Can you work these out from the model? Positions are in its coordinate system, mm. A direction names the side the tool comes from. Give positions to 0.01 mm unless a question says otherwise; leave off trailing zeros. Loops run counter-clockwise (first coordinate to the right, second up) from the corner with the lowest first, then second, coordinate; pieces in that order, holes last. Notation, with made-up numbers: (84.25, 3) - (98.25, 3) arc R16 ccw to (98.25, 15) - close; hole circle Ø3 at (10, 80.5). An arc over 180 degrees is marked (long way). Answer as a JSON object with one key per item and string values. Group by question number.
Item 1: Suppose I cut it at D-D on z = -18.5. Write out the boundary of the cut face in (x, y).
Item 2: Thinking about a two-plate mould opening in Y: for faces 3 (the flat face through (50, 16.8, -5)), 4 (the cylindrical face through (50.089, 9.937, -2.367)), 5 (the flat face through (50, 18, -9.525)), which applies, pulls with the +Y half, pulls with the -Y half, needs draft (parallel to the pull), parting line crosses it, or undercut?
Item 3: Please list where these lines run through material, in increasing order: L1, parallel to X at y = 10, z = -5; L2, parallel to Y at x = 23.5, z = -5; L3, parallel to Z at x = 82.55, y = 13.5.
Item 4: Suppose I cut it at B-B on x = 23.5. Write out the boundary of the cut face in (y, z) (3 decimals), and give its area (3 significant figures).
Item 5: Which directions (+Z, -Z, +X, -X, +Y, -Y) give clear straight access to the entire face, cutting with the end or side of a thin tool? Please do faces 1 (the flat face through (50, 3.2, -5)), 2 (the cylindrical face through (84.075, 10.095, -4.13)).
Item 6: Suppose I cut it at C-C on y = 15. Write out the boundary of the cut face in (x, z), and give its area (3 significant figures).
Item 7: Will these pins go through, and if not, where does the flat tip stop? pin 1 (2 mm diameter, centred on x = 54, y = 10, fed in from +Z); pin 2 (1.6 mm diameter, centred on x = 36.5, y = 18, fed in from +Z) (3 decimals); pin 3 (10.5 mm diameter, centred on x = 29, z = -4, fed in from +Y).
from build123d import *

# Parameters (mm, degrees)
BOSS_EXTRUDE1_DEPTH = 101.6
CUT_EXTRUDE2_DEPTH  = 101.6
SKETCH5_R           = 1.651
CUT_EXTRUDE3_DEPTH  = 13.5992
FILLET1_R           = 2.54


with BuildPart() as part:
    # Sketch1 → Boss-Extrude1 (new body)
    with BuildSketch(Plane(origin=(0, 0, 0), x_dir=(0, 0, -1), z_dir=(1, 0, 0))):
        with BuildLine():
            Line((0, 16.7996), (0, 3.2004))
            Line((0, 3.2004), (9.525, 3.2004))
            Line((9.525, 3.2004), (9.525, 0))
            Line((9.525, 0), (9.672001208, 0))
            ThreePointArc((9.672001208, 0), (12.1043061, 0.647018058), (13.89365381, 2.417039025))
            Line((13.89365381, 2.417039025), (24.215623453, 20))
            Line((24.215623453, 20), (9.525, 20))
            Line((9.525, 20), (9.525, 16.7996))
            Line((9.525, 16.7996), (0, 16.7996))
        make_face()
    extrude(amount=BOSS_EXTRUDE1_DEPTH)

    # Sketch4 → Cut-Extrude2 (cut)
    with BuildSketch(Plane.ZY):
        with BuildLine():
            Line((0, 13.526281186), (0, 6.473718814))
            ThreePointArc((0, 6.473718814), (-2.36728, 10), (0, 13.526281186))
        make_face()
    extrude(amount=-CUT_EXTRUDE2_DEPTH, mode=Mode.SUBTRACT)

    # Sketch5 → Cut-Extrude3 (cut)
    with BuildSketch(Plane(origin=(0, 16.7996, 0), x_dir=(1, 0, 0), z_dir=(0, 1, 0))):
        with Locations((19.05, 4.7625)):
            Circle(SKETCH5_R)
        with Locations((82.55, 4.7625)):
            Circle(SKETCH5_R)
    extrude(amount=-CUT_EXTRUDE3_DEPTH, mode=Mode.SUBTRACT)

    # Fillet1
    fillet1_edges = [part.edges().sort_by_distance(p)[0] for p in [
        (50.8, 20, -24.215623453),
    ]]
    fillet(fillet1_edges, radius=FILLET1_R)


solid = part.part
Worked out:
{
 "1": {"outline": "(0, 10.26) - (101.6, 10.26) - (101.6, 20) - (0, 20) - close"},
 "2": {"face 3": "pulls with the +Y half", "face 4": "undercut", "face 5": "needs draft"},
 "3": {"L1": "x = 0 to 17.42, 20.68 to 80.92, 84.18 to 101.6", "L2": "y = 3.2 to 16.8", "L3": "z = -20.4 to -6.41, -3.11 to -0.06"},
 "4": {"outline": "(0, -9.672) arc R4.895 ccw to (2.417, -13.894) - (16.174, -21.97) arc R2.54 ccw to (20, -19.779) - (20, -9.525) - (16.8, -9.525) - (16.8, 0) - (13.526, 0) arc R3.81 cw to (6.474, 0) - (3.2, 0) - (3.2, -9.525) - (0, -9.525) - close", "area": "288 mm2"},
 "5": {"face 1": "+Z, +X, -X, -Y", "face 2": "+Y, -Y"},
 "6": {"outline": "(0, -21.28) - (101.6, -21.28) - (101.6, 0) - (0, 0) - close; hole circle Ø3.3 at (19.05, -4.76); hole circle Ø3.3 at (82.55, -4.76)", "area": "2,140 mm2"},
 "7": {"pin 1": "stops at z = -2.23", "pin 2": "stops at z = -9.525", "pin 3": "stops at y = 16.8"}
}
